```python
from build123d import *

# Parameters (mm, degrees)
F0_W     = 30
F0_H     = 6
F1_DEPTH = 100
F2_R     = 1.025
F3_DEPTH = 6
F4_W     = 3
F4_H     = 50
F5_DEPTH = 30
F6_W     = 4.600006
F6_H     = 4.600006
F6_W_2   = 4.6
F6_H_2   = 4.6
F6_W_3   = 4.600004
F6_H_3   = 4.600004
F7_DEPTH = 3
F8_R     = 2.5
F9_DEPTH = 4.1


with BuildPart() as f1:
    # F0 (on Top) → F1 (new body)
    with BuildSketch(Plane.XY):
        Rectangle(F0_W, F0_H)
    extrude(amount=F1_DEPTH)

    # F2 (on face) → F3 (cut, through all)
    with BuildSketch(Plane.XZ.offset(3)):
        with Locations((11, 4.025)):
            Circle(F2_R)
        with Locations((11, 44.025)):
            Circle(F2_R)
        with Locations((-11, 44.025)):
            Circle(F2_R)
        with Locations((-11, 4.025)):
            Circle(F2_R)
    extrude(amount=-F3_DEPTH, mode=Mode.SUBTRACT)

    # F4 (on face) → F5 (cut, through all)
    with BuildSketch(Plane.YZ.offset(15)):
        with Locations((1.5, 75)):
            Rectangle(F4_W, F4_H)
    extrude(amount=-F5_DEPTH, mode=Mode.SUBTRACT)

    # F6 (on face) → F7 (join)
    with BuildSketch(Plane(origin=(0, 0, 0), x_dir=(-1, 0, 0), z_dir=(0, 1, 0))):
        with Locations((-7.5, 92.5)):
            Rectangle(F6_W, F6_H)
        with Locations((7.5, 92.5)):
            Rectangle(F6_W, F6_H)
        with Locations((-7.5, 62.5)):
            Rectangle(F6_W_2, F6_H_2)
        with Locations((7.5, 62.5)):
            Rectangle(F6_W_3, F6_H_3)
    extrude(amount=F7_DEPTH)

    # F8 (on face) → F9 (cut)
    with BuildSketch(Plane(origin=(0, 3, 0), x_dir=(-1, 0, 0), z_dir=(0, 1, 0))):
        with Locations((11, 44.025)):
            Circle(F8_R)
        with Locations((-11, 44.025)):
            Circle(F8_R)
        with Locations((-11, 4.025)):
            Circle(F8_R)
        with Locations((11, 4.025)):
            Circle(F8_R)
    extrude(amount=-F9_DEPTH, mode=Mode.SUBTRACT)


solid = f1.part
```
Here's how the part is built. I have some questions about the finished solid (model axes, mm). A direction names the side the tool comes from. Coordinates: 2 decimals unless noted, no trailing zeros. Order: outer loops, then holes, each group sorted by start corner. A loop starts at its lowest first (then second) coordinate and runs counter-clockwise, first axis right, second up. Notation, with made-up numbers: (-25.75, -36.5) -> (5.25, -36.5) arc R22 cw to (5.25, -23.5) -> close; hole circle Ø7 at (4, 36). An arc over 180 degrees is marked (long way). Return JSON: item names as keys, results as strings.
1) If I drill on probe 1 along Z at (x, y) = (11, -2.6); probe 2 along Z at (x, y) = (6.5, 1.7); probe 3 along X at (y, z) = (2.25, 61), over which ranges is the centre line in solid material (lowest first)?
Conclusion:
{"probe 1": "z = 0 to 3, 5.05 to 43, 45.05 to 100", "probe 2": "z = 0 to 50, 60.2 to 64.8, 90.2 to 94.8", "probe 3": "x = -9.8 to -5.2, 5.2 to 9.8"}
2) On a 3-axis mill with a long thin cutter (end or side, diameter ignored), from which of +Z, -Z, +X, -X, +Y, -Y can I reach the whole of each face in a straight line? I mean faces 1 (the flat face through (-5.2, 1, 92)), 2 (the flat face through (-9.8, 1, 62)), 3 (the flat face through (0, 1, 50)), 4 (the cylindrical face through (-8.5, 1, 4.1)). Say none if no direction works.
Conclusion:
{"face 1": "+Z, +Y", "face 2": "+Z, -X, +Y", "face 3": "+X, -X, +Y", "face 4": "+Y"}
3) Thinking about a two-plate mould opening in Z: for faces 5 (the flat face through (-7, 3, 63)), 6 (the flat face through (10, -1.1, 3)), 7 (the flat face through (0, -1, 100)), 8 (the flat face through (-7, 1, 64.8)), which applies, +Z half, -Z half, draft (parallel to the pull), parting line (faces both ways), or undercut?
Conclusion:
{"face 5": "draft", "face 6": "undercut", "face 7": "+Z half", "face 8": "undercut"}
4) I'm going to push flat-ended pins straight in: P1, Ø2.5, axis at x = 8, y = 2, coming from the -Z side; P2, Ø1.5, axis at y = 1.5, z = 62, coming from the -X side; P3, Ø3, axis at x = -11, z = 44.025, coming from the +Y side; P4, Ø1.5, axis at y = 1.5, z = 62.5, coming from the +X side. Where does each tip first touch, or does it pass through?
Conclusion:
{"P1": "stops at z = 0", "P2": "stops at x = -9.8", "P3": "stops at y = -1.1", "P4": "stops at x = 9.8"}
5) If we section it at B-B on y = 1.55: State how many separate pieces and enclosed holes the cut face has, plus the area to 3 significant figures.
Conclusion:
{"separate pieces": "5", "enclosed holes": "4", "area": "1,510 mm²"}
6) If we section it at C-C on x = 3.5: List the corners of the cut face in (y, z) for me.
Conclusion:
{"outline": "(-3, 0) -> (3, 0) -> (3, 50) -> (0, 50) -> (0, 100) -> (-3, 100) -> close"}
7) If we section it at A-A on x = 11: List the corners of the cut face in (y, z) for me (3 decimals), plus the area to 3 significant figures.
Conclusion:
{"outline": "(-3, 0) -> (3, 0) -> (3, 1.525) -> (-1.1, 1.525) -> (-1.1, 3) -> (-3, 3) -> close; (-3, 5.05) -> (-1.1, 5.05) -> (-1.1, 6.525) -> (3, 6.525) -> (3, 41.525) -> (-1.1, 41.525) -> (-1.1, 43) -> (-3, 43) -> close; (-3, 45.05) -> (-1.1, 45.05) -> (-1.1, 46.525) -> (3, 46.525) -> (3, 50) -> (0, 50) -> (0, 100) -> (-3, 100) -> close", "area": "401 mm²"}
